from build123d import *

# Parameters (mm, degrees)
SKETCH1_W           = 1000
SKETCH1_H           = 195
BOSS_EXTRUDE1_DEPTH = 1000
SKETCH2_R           = 50
SKETCH2_R_2         = 40
SKETCH2_R_3         = 38.049771674
BOSS_EXTRUDE2_DEPTH = 100
CUT_EXTRUDE1_START  = -964
SKETCH5_R           = 40
SKETCH5_R_2         = 38.049771674
CUT_EXTRUDE1_DEPTH  = 964


with BuildPart() as part:
    # Sketch1 → Boss-Extrude1 (new body)
    with BuildSketch(Plane.XY):
        with Locations((500, -97.5)):
            Rectangle(SKETCH1_W, SKETCH1_H)
    extrude(amount=BOSS_EXTRUDE1_DEPTH)

    # Sketch2 → Boss-Extrude2 (add)
    # profile 1 of 4: a face of its own
    with BuildSketch(Plane.XY.offset(1000)):
        with Locations(Location((100, -97.5, 0), (0, 0, 180))):
            Circle(SKETCH2_R)
        with Locations((100, -97.5)):
            Circle(SKETCH2_R_2, mode=Mode.SUBTRACT)
    # profile 2 of 4: a face of its own
    with BuildSketch(Plane.XY.offset(1000)):
        with Locations(Location((300, -97.5, 0), (0, 0, 180))):
            Circle(SKETCH2_R)
        with Locations((300, -97.5)):
            Circle(SKETCH2_R_3, mode=Mode.SUBTRACT)
    # profile 3 of 4: a face of its own
    with BuildSketch(Plane.XY.offset(1000)):
        with Locations(Location((700, -97.5, 0), (0, 0, 180))):
            Circle(SKETCH2_R)
        with Locations((700, -97.5)):
            Circle(SKETCH2_R_2, mode=Mode.SUBTRACT)
    # profile 4 of 4: a face of its own
    with BuildSketch(Plane.XY.offset(1000)):
        with Locations(Location((900, -97.5, 0), (0, 0, 180))):
            Circle(SKETCH2_R)
        with Locations((900, -97.5)):
            Circle(SKETCH2_R_2, mode=Mode.SUBTRACT)
    extrude(amount=BOSS_EXTRUDE2_DEPTH)

    # Sketch5 → Cut-Extrude1 (cut)
    with BuildSketch(Plane.XY.offset(1000).offset(CUT_EXTRUDE1_START)):
        with Locations((100, -97.5)):
            Circle(SKETCH5_R)
        with Locations((300, -97.5)):
            Circle(SKETCH5_R_2)
        with Locations((700, -97.5)):
            Circle(SKETCH5_R)
        with Locations((900, -97.5)):
            Circle(SKETCH5_R)
    extrude(amount=CUT_EXTRUDE1_DEPTH, mode=Mode.SUBTRACT)


solid = part.part
Geometry: final body of the model. Coordinates: model frame, mm. A direction names the side the tool comes from. Round coordinates to 2 decimals unless told otherwise and drop trailing zeros. Loops run counter-clockwise (first coordinate to the right, second up) from the corner with the lowest first, then second, coordinate; pieces in that order, holes last.
Q1. Section B-B on x = 300. Return loops of the section in (y, z).
Q2. Section A-A on z = 714.5. Return loops of the section in (x, y).
Q3. Material intervals for L1, parallel to X at y = -97, z = 576; L2, parallel to X at y = -102, z = 790; L3, parallel to Y at x = 700, z = 544, sorted ascending.
Q4. Section C-C on y = -178. Return loops of the section in (x, z).
Q5. Pin query (flat end, axial travel): P1, Ø10, axis at x = 348.5, y = -84, coming from the -Z side; P2, Ø24, axis at x = 882, y = -78, coming from the +Z side. Return the tip coordinate at first contact, or that it passes through.
Q6. Section D-D on x = 100. Return loops of the section in (y, z).
Q7. Pull-direction query (Y, two-part tool) for faces 3 (the cylindrical face through (736.95, -112.82, 560.55)), 4 (the flat face through (122.5, -131.1, 1100)), 5 (the cylindrical face through (652.31, -112.52, 1049.3)); classes: released by +Y, released by -Y, zero draft, split by the parting line, or undercut.
Q8. Access query for faces 1 (the flat face through (493, -96, 0)), 2 (the cylindrical face through (138.153, -85.485, 560.552)). Directions: +Z, -Z, +X, -X, +Y, -Y. A direction counts if a zero-diameter tool reaches every point of the face in a straight line with its end or side. Return the directions, or none.
Evaluation:
1. outline: (-195, 0) - (0, 0) - (0, 1000) - (-47.5, 1000) - (-47.5, 1100) - (-59.45, 1100) - (-59.45, 36) - (-135.55, 36) - (-135.55, 1100) - (-147.5, 1100) - (-147.5, 1000) - (-195, 1000) - close
2. outline: (0, -195) - (1000, -195) - (1000, 0) - (0, 0) - close; hole circle Ø80 at (100, -97.5); hole circle Ø76.1 at (300, -97.5); hole circle Ø80 at (700, -97.5); hole circle Ø80 at (900, -97.5)
3. L1: x = 0 to 60, 140 to 261.95, 338.05 to 660, 740 to 860, 940 to 1000
3. L2: x = 0 to 60.25, 139.75 to 262.22, 337.78 to 660.25, 739.75 to 860.25, 939.75 to 1000
3. L3: y = -195 to -137.5, -57.5 to 0
4. outline: (0, 0) - (1000, 0) - (1000, 1000) - (0, 1000) - close
5. P1: stops at z = 0
5. P2: stops at z = 36
6. outline: (-195, 0) - (0, 0) - (0, 1000) - (-47.5, 1000) - (-47.5, 1100) - (-57.5, 1100) - (-57.5, 36) - (-137.5, 36) - (-137.5, 1100) - (-147.5, 1100) - (-147.5, 1000) - (-195, 1000) - close
7. face 3: undercut
7. face 4: zero draft
7. face 5: split by the parting line
8. face 1: -Z, +X, -X, +Y, -Y
8. face 2: +Z
